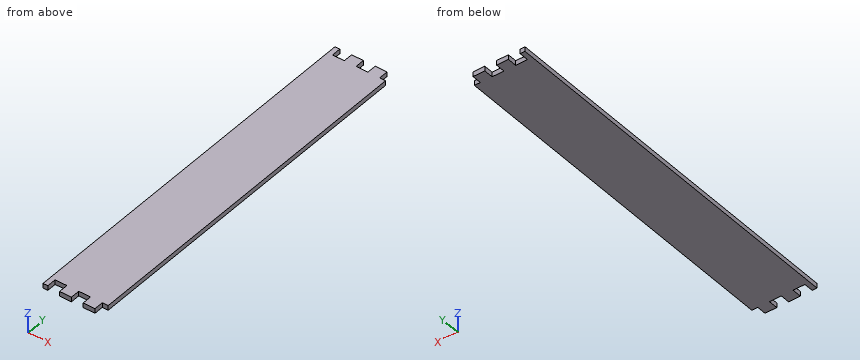
from build123d import *

# Parameters (mm, degrees)
F1_DEPTH = 2
F3_DEPTH = 5
F4_W     = 28.972704
F4_H     = 205.101743
F5_DEPTH = 25


with BuildPart() as f1:
    # F0 (on Top) → F1 (new body)
    with BuildSketch(Plane.XY):
        Polygon((-24.541279, -80), (0, -80), (24.541279, -80), (24.541279, 0), (24.541279, 80), (0, 80), (-24.541279, 80), (-24.541279, 0), align=None)
    extrude(amount=F1_DEPTH)

    # F2 (on face) → F3 (cut)
    with BuildSketch(Plane.XY.offset(2)):
        Polygon((2.5, -76), (0, -76), (-2.5, -76), (-2.5, -80), (-7.5, -80), (-7.5, -76), (-12.5, -76), (-12.5, -80), (-17.5, -80), (-17.5, -76), (-22.5, -76), (-22.5, -80), (-22.5, -83.697788), (22.5, -83.697788), (22.5, -80), (22.5, -76), (17.5, -76), (17.5, -80), (12.5, -80), (12.5, -76), (7.5, -76), (7.5, -80), (2.5, -80), align=None)
        Polygon((-22.5, 80), (-22.5, 76), (-17.5, 76), (-17.5, 80), (-12.5, 80), (-12.5, 76), (-7.5, 76), (-7.5, 80), (-2.5, 80), (-2.5, 76), (0, 76), (2.5, 76), (2.5, 80), (7.5, 80), (7.5, 76), (12.5, 76), (12.5, 80), (17.5, 80), (17.5, 76), (22.5, 76), (22.5, 80), (22.5, 83.697788), (-22.5, 83.697788), align=None)
    extrude(amount=-F3_DEPTH, mode=Mode.SUBTRACT)

    # F4 (on face) → F5 (cut)
    with BuildSketch(Plane.XY.offset(2)):
        with Locations((14.486352, 8.12903)):
            Rectangle(F4_W, F4_H)
    extrude(amount=-F5_DEPTH, mode=Mode.SUBTRACT)


solid = f1.part
Build history of the part. All positions in model axes, mm. Round coordinates to 2 decimals unless told otherwise and drop trailing zeros. Write each loop counter-clockwise with the first axis right and the second up, starting at its lowest first coordinate (ties: lowest second). Pieces come first, ordered by that corner, then holes. Notation, with made-up numbers: (53, 44.25) - (72, 44.25) arc R32 ccw to (72, 73.25) - close; hole circle Ø2 at (3.5, 43.5). An arc over 180 degrees is marked (long way). One line per question, with ' | ' between items.
1. Band-saw the part on A-A, the plane z = 1.45. Write the cut outline in (x, y).
Results are:
outline: (-24.54, -80) - (-22.5, -80) - (-22.5, -76) - (-17.5, -76) - (-17.5, -80) - (-12.5, -80) - (-12.5, -76) - (-7.5, -76) - (-7.5, -80) - (-2.5, -80) - (-2.5, -76) - (0, -76) - (0, 76) - (-2.5, 76) - (-2.5, 80) - (-7.5, 80) - (-7.5, 76) - (-12.5, 76) - (-12.5, 80) - (-17.5, 80) - (-17.5, 76) - (-22.5, 76) - (-22.5, 80) - (-24.54, 80) - close
2. Drop flat-ended pins along their axis: pin 1 Ø0.6 at (y, z) = (-78.5, 0.5) entering from +X; pin 2 Ø0.6 at (x, z) = (-20, 0.5) entering from -Y. Give the stop position or say it passes through.
Results are:
pin 1: x = -2.5 | pin 2: y = -76
3. Drill centre line: line 1 along Y through (x, z) = (-20.5, 0.2). Where is it in solid material? Low to high. Write a range as from..to.
Results are:
line 1: -76..76
4. Band-saw the part on B-B, the plane x = -19. Write the cut outline in (y, z).
Results are:
outline: (-76, 0) - (76, 0) - (76, 2) - (-76, 2) - close
